```python
from build123d import *

# Parameters (mm, degrees)
SKETCH1_W           = 4.6228
SKETCH1_H           = 4.819787269
SKETCH1_H_2         = 4.6228
BOSS_EXTRUDE1_DEPTH = 6.35
FILLET2_R           = 3.175
FILLET3_R           = 3.175


with BuildPart() as part:
    # Sketch1 → Boss-Extrude1 (new body)
    with BuildSketch(Plane(origin=(0, 0, 0), x_dir=(1, 0, 0), z_dir=(0, 1, 0))):
        Polygon((0, 0), (254, 0), (254, -76.2), (190.5, -76.2), (190.5, -25.4), (0, -25.4), align=None)
        with Locations((6.522414475, -19.224693634)):
            Rectangle(SKETCH1_W, SKETCH1_H, mode=Mode.SUBTRACT)
        with Locations((6.3754, -6.3754)):
            Rectangle(SKETCH1_W, SKETCH1_H_2, mode=Mode.SUBTRACT)
        with Locations((69.8754, -6.3754)):
            Rectangle(SKETCH1_W, SKETCH1_H_2, mode=Mode.SUBTRACT)
        with Locations((70.022414475, -19.224693634)):
            Rectangle(SKETCH1_W, SKETCH1_H, mode=Mode.SUBTRACT)
        with Locations((196.8754, -6.3754)):
            Rectangle(SKETCH1_W, SKETCH1_H_2, mode=Mode.SUBTRACT)
        with Locations((247.822414475, -31.974693634)):
            Rectangle(SKETCH1_W, SKETCH1_H, mode=Mode.SUBTRACT)
        with Locations((247.822414475, -44.724693634)):
            Rectangle(SKETCH1_W, SKETCH1_H, mode=Mode.SUBTRACT)
        with Locations((247.822414475, -57.474693634)):
            Rectangle(SKETCH1_W, SKETCH1_H, mode=Mode.SUBTRACT)
        with Locations((209.722414475, -31.8762)):
            Rectangle(SKETCH1_W, SKETCH1_H_2, mode=Mode.SUBTRACT)
        with Locations((209.722414475, -44.6262)):
            Rectangle(SKETCH1_W, SKETCH1_H_2, mode=Mode.SUBTRACT)
        with Locations((209.722414475, -57.3762)):
            Rectangle(SKETCH1_W, SKETCH1_H_2, mode=Mode.SUBTRACT)
    extrude(amount=BOSS_EXTRUDE1_DEPTH)

    # Fillet2
    fillet2_edges = [part.edges().sort_by_distance(p)[0] for p in [
        (0, 3.175, 25.4),
    ]]
    fillet(fillet2_edges, radius=FILLET2_R)

    # Fillet3
    fillet3_edges = [part.edges().sort_by_distance(p)[0] for p in [
        (0, 3.175, 0),
        (254, 3.175, 0),
        (254, 3.175, 76.2),
        (190.5, 3.175, 76.2),
    ]]
    fillet(fillet3_edges, radius=FILLET3_R)


solid = part.part
```
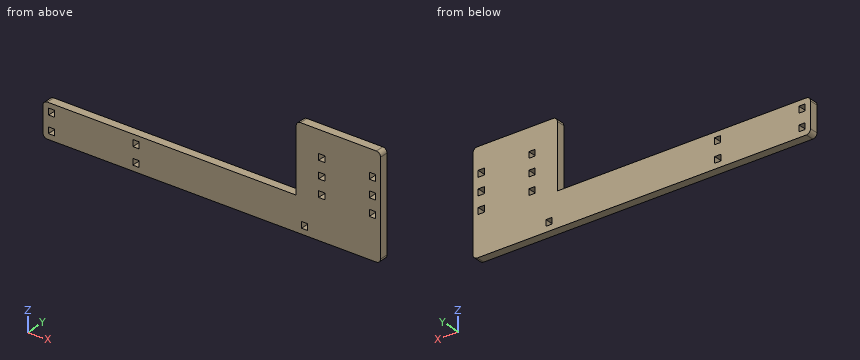
Can you work these out from the model? Positions are in its coordinate system, mm. Coordinates: 2 decimals unless noted, no trailing zeros. Loops run counter-clockwise (first coordinate to the right, second up) from the corner with the lowest first, then second, coordinate; pieces in that order, holes last.
Item 1: Suppose I cut it at B-B (x = 137). Please give me the cut outline in (y, z).
Answers below:
outline: (0, 0) - (6.35, 0) - (6.35, 25.4) - (0, 25.4) - close
Item 2: Suppose I cut it at A-A (y = 2.75). State how many separate pieces and enclosed holes the cut face has, then the cut area to 3 significant figures.
Answers below:
separate pieces: 1
enclosed holes: 11
area: 9,430 mm2
Item 3: Please list where these lines run through material, in increasing order: L1, parallel to X at y = 4, z = 44.5; L2, parallel to X at y = 4.5, z = 19; L3, parallel to X at y = 2.25, z = 35.5.
Answers below:
L1: x = 190.5 to 207.41, 212.03 to 245.51, 250.13 to 254
L2: x = 0 to 4.21, 8.83 to 67.71, 72.33 to 254
L3: x = 190.5 to 254
Item 4: Suppose I cut it at C-C (z = 49.5). Please give me the cut outline in (x, y).
Answers below:
outline: (190.5, 0) - (254, 0) - (254, 6.35) - (190.5, 6.35) - close
Item 5: I'm going to push flat-ended pins straight in: pin 1 (1.4 mm diameter, centred on x = 69, y = 4.5, fed in from +Z); pin 2 (3.5 mm diameter, centred on y = 3, z = 57.5, fed in from -X). Where does each tip first touch, or does it pass through?
Answers below:
pin 1: stops at z = 25.4
pin 2: stops at x = 190.5
